Here's how the part is built. I have some questions about the finished solid (model axes, mm). A direction names the side the tool comes from. Give positions to 0.01 mm unless a question says otherwise; leave off trailing zeros. Order: outer loops, then holes, each group sorted by start corner. A loop starts at its lowest first (then second) coordinate and runs counter-clockwise, first axis right, second up. Notation, with made-up numbers: (52.25, 44.5) -> (95.25, 44.5) arc R6 cw to (95.25, 51.5) -> close; hole circle Ø6 at (76, 50.25). An arc over 180 degrees is marked (long way). Write each question's results on one line, items separated by ' | '. Start each with the question number.
Q1. I need wall thicknesses on line 1 along Y through (x, z) = (43, 9.5); line 2 along X through (y, z) = (13.75, 4.5); line 3 along X through (y, z) = (13.25, 9.5). Which ranges of each line are inside material? Lowest first, please. Write a range as [from, to].
Q2. Thinking about a two-plate mould opening in X: for faces 4 (the face through (26, 15, 6)), 5 (the face through (47, 23.57, 10.46)), 6 (the face through (24, 3, -18)), which applies, pulls with the +X half, pulls with the -X half, needs draft (parallel to the pull), parting line crosses it, or undercut?
Q3. Imagine slicing it at C-C, the plane z = -3.5. Please give me the cut outline in (x, y).
Q4. Imagine slicing it at A-A, the plane y = 12.5. Please give me the cut outline in (x, z), then the cut area to 3 significant figures.
Q5. Imagine slicing it at D-D, the plane x = 13. Please give me the cut outline in (y, z).
Q6. I'm going to push flat-ended pins straight in: pin 1 (1.7 mm diameter, centred on y = 2, z = -17, fed in from -X); pin 2 (4 mm diameter, centred on x = 27.5, y = 12, fed in from -Z); pin 3 (6.5 mm diameter, centred on x = 43.5, y = 13, fed in from -Z); pin 4 (1.5 mm diameter, centred on x = -11, z = 6, fed in from +Y). Where does each tip first touch, or does it pass through?
Q7. For faces 1 (the face through (0, 15, 7)), 2 (the face through (-14, 12, 8)), 3 (the face through (26, 2, -17)), which set-ups out of +Z, -Z, +X, -X, +Y, -Y let a thin tool reach every point of the face, with its end or its side?
Q8. Imagine slicing it at B-B, the plane y = 6. Please give me the cut outline in (x, z).
```python
from build123d import *

# Parameters (mm, degrees)
BOSS_EXTRUDE1_DEPTH = 25
SKETCH4_R           = 1.75
CUT_EXTRUDE1_DEPTH  = 6
FILLET1_R           = 5
FILLET2_R           = 2
SKETCH5_W           = 26
SKETCH5_H           = 5
BOSS_EXTRUDE2_DEPTH = 31


with BuildPart() as part:
    # Sketch1 → Boss-Extrude1 (new body)
    with BuildSketch(Plane(origin=(0, 0, 0), x_dir=(1, 0, 0), z_dir=(0, 1, 0))):
        with BuildLine():
            Line((-7.5, 0), (-7.5, -8))
            Line((-7.5, -8), (-22.5, -8))
            Line((-22.5, -8), (-22.5, -13))
            Line((-22.5, -13), (0, -13))
            Line((0, -13), (0, 0))
            ThreePointArc((0, 0), (13, 13), (26, 0))
            Line((26, 0), (26, -13))
            Line((26, -13), (48.5, -13))
            Line((48.5, -13), (48.5, -8))
            Line((48.5, -8), (33.5, -8))
            Line((33.5, -8), (33.5, 0))
            ThreePointArc((33.5, 0), (13, 20.5), (-7.5, 0))
        make_face()
    extrude(amount=BOSS_EXTRUDE1_DEPTH)

    # Sketch4 → Cut-Extrude1 (cut, through all)
    with BuildSketch(Plane(origin=(0, 0, 8), x_dir=(-1, 0, 0), z_dir=(0, 0, -1))):
        with Locations((-43, 12.5)):
            Circle(SKETCH4_R)
        with Locations((17, 12.5)):
            Circle(SKETCH4_R)
    extrude(amount=-CUT_EXTRUDE1_DEPTH, mode=Mode.SUBTRACT)

    # Fillet1
    fillet1_edges = [part.edges().sort_by_distance(p)[0] for p in [
        (-22.5, 0, 10.5),
        (48.5, 0, 10.5),
        (48.5, 25, 10.5),
        (-22.5, 25, 10.5),
    ]]
    fillet(fillet1_edges, radius=FILLET1_R)

    # Fillet2
    fillet2_edges = [part.edges().sort_by_distance(p)[0] for p in [
        (-7.5, 12.5, 8),
        (33.5, 12.5, 8),
    ]]
    fillet(fillet2_edges, radius=FILLET2_R)

    # Sketch5 → Boss-Extrude2 (add)
    with BuildSketch(Plane.XY.offset(13)):
        with Locations((13, 2.5)):
            Rectangle(SKETCH5_W, SKETCH5_H)
    extrude(amount=-BOSS_EXTRUDE2_DEPTH)


solid = part.part
```
Geometry check:
1) line 1: [0, 10.75], [14.25, 25] | line 2: [-7.5, 0], [26, 33.5] | line 3: [-22.5, -18.58], [-15.42, 0], [26, 41.42], [44.58, 48.5]
2) face 4: undercut | face 5: pulls with the +X half | face 6: needs draft
3) outline: (-7.2, 0) -> (33.2, 0) -> (33.2, 25) -> (25.52, 25) -> (25.52, 5) -> (0.48, 5) -> (0.48, 25) -> (-7.2, 25) -> close
4) outline: (-22.5, 8) -> (-18.75, 8) -> (-18.75, 13) -> (-22.5, 13) -> close; (-15.25, 8) -> (-9.5, 8) arc R2 cw to (-7.5, 6) -> (-7.5, 0) arc R20.5 ccw to (33.5, 0) -> (33.5, 6) arc R2 cw to (35.5, 8) -> (41.25, 8) -> (41.25, 13) -> (26, 13) -> (26, 0) arc R13 cw to (0, 0) -> (0, 13) -> (-15.25, 13) -> close; (44.75, 8) -> (48.5, 8) -> (48.5, 13) -> (44.75, 13) -> close | area: 706 mm²
5) outline: (0, -20.5) -> (25, -20.5) -> (25, -13) -> (5, -13) -> (5, 13) -> (0, 13) -> close
6) pin 1: x = 0 | pin 2: z = -16.25 | pin 3: z = 8 | pin 4: through
7) face 1: +Z, +Y | face 2: -Z, -X, +Y, -Y | face 3: -Z, +X, +Y, -Y
8) outline: (-22.5, 8) -> (-9.5, 8) arc R2 cw to (-7.5, 6) -> (-7.5, 0) arc R20.5 ccw to (33.5, 0) -> (33.5, 6) arc R2 cw to (35.5, 8) -> (48.5, 8) -> (48.5, 13) -> (26, 13) -> (26, 0) arc R13 cw to (0, 0) -> (0, 13) -> (-22.5, 13) -> close
